Geometry check sheet. Reference: drawing and pictorial views, mm from the part's lowest x, y, z. A direction names the side the tool comes from. Round coordinates to 2 decimals unless told otherwise and drop trailing zeros. Write each loop counter-clockwise with the first axis right and the second up, starting at its lowest first coordinate (ties: lowest second). Pieces come first, ordered by that corner, then holes. Notation, with made-up numbers: (14, -33) -> (65, -33) arc R22 cw to (65, -2) -> close; hole circle Ø11 at (58.5, 53). An arc over 180 degrees is marked (long way). Answer as a JSON object with one key per item and string values. Group by question number.
(1) Sectioned sample at B-B on y = 19.05. Record the cut outline in (x, z).
(2) Set-up check for the marked faces 1, 2 and 3: record each of +Z, -Z, +X, -X, +Y, -Y from which the full face is reachable in a straight line by a thin tool's end or side.
(3) Scan lines: L1, parallel to X at y = 8, z = 8 (1 decimal); L2, parallel to Y at x = 5, z = 30 (1 decimal); L3, parallel to Y at x = 5.5, z = 27.5. Record each from-to range of solid material in increasing order. Write a range as from..to.
(4) Gauge pin test, flat ends, axial feed: pin 1 Ø4.5 at (y, z) = (4.5, 28) entering from +X (1 decimal); pin 2 Ø2 at (y, z) = (6.06, 41.02) entering from -X; pin 3 Ø2.5 at (x, z) = (7, 23.5) entering from +Y; pin 4 Ø3 at (y, z) = (26, 19) entering from +X. Record the tip position at first contact, or that the pin passes through.
(5) Sectioned sample at D-D on y = 31. Record the cut outline in (x, z) (1 decimal).
(6) Sectioned sample at C-C on x = 6.75. Record the cut outline in (y, z) (1 decimal), and give its area (3 significant figures).
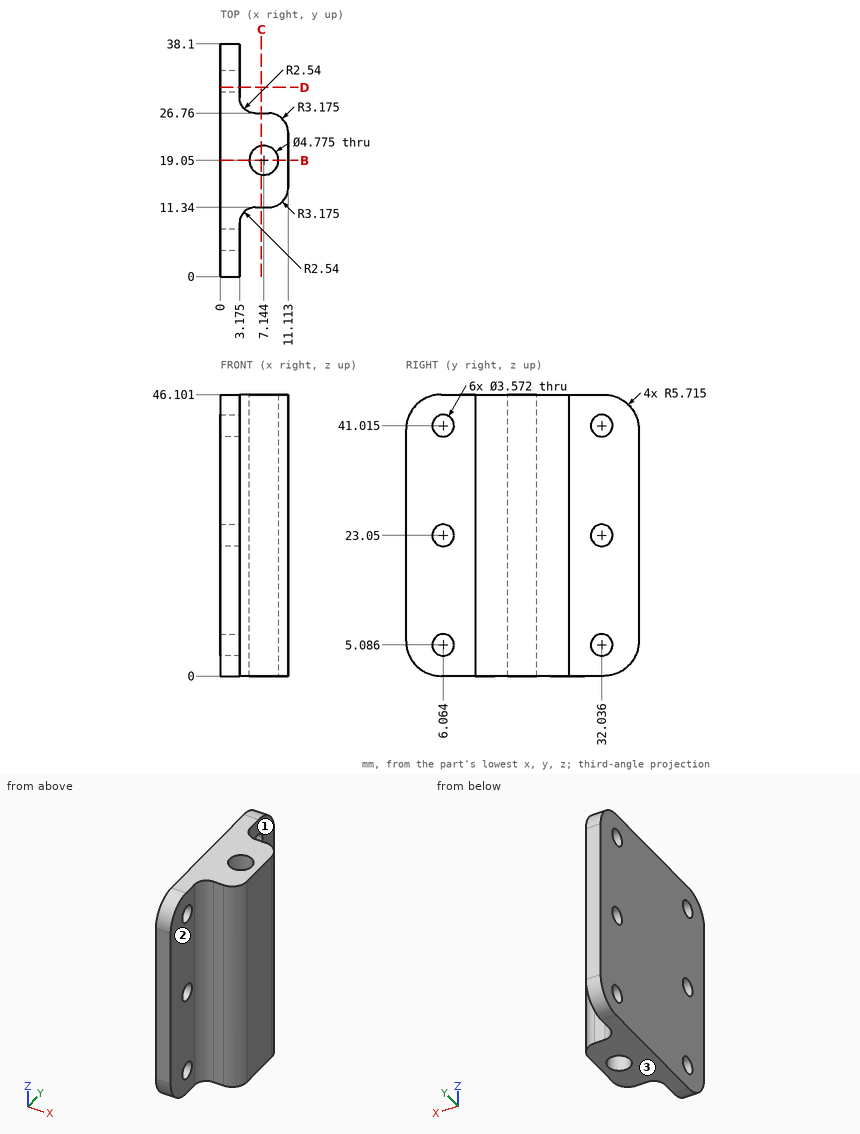
Computed values:
{
 "1": {"outline": "(0, 0) -> (4.76, 0) -> (4.76, 46.1) -> (0, 46.1) -> close; (9.53, 0) -> (11.11, 0) -> (11.11, 46.1) -> (9.53, 46.1) -> close"},
 "2": {"face 1": "+Z, -Z, +X, +Y", "face 2": "+Z, -Z, +X, -Y", "face 3": "-Z, +X, -X, +Y, -Y"},
 "3": {"L1": "0..3.2", "L2": "11.2..18, 20.1..26.9", "L3": "11.33..17.32, 20.78..26.77"},
 "4": {"pin 1": "x = 3.2", "pin 2": "through", "pin 3": "y = 26.76", "pin 4": "x = 10.98"},
 "5": {"outline": "(0, 0) -> (3.2, 0) -> (3.2, 3.6) -> (0, 3.6) -> close; (0, 6.5) -> (3.2, 6.5) -> (3.2, 21.6) -> (0, 21.6) -> close; (0, 24.5) -> (3.2, 24.5) -> (3.2, 39.6) -> (0, 39.6) -> close; (0, 42.5) -> (3.2, 42.5) -> (3.2, 46.1) -> (0, 46.1) -> close"},
 "6": {"outline": "(11.3, 0) -> (16.7, 0) -> (16.7, 46.1) -> (11.3, 46.1) -> close; (21.4, 0) -> (26.8, 0) -> (26.8, 46.1) -> (21.4, 46.1) -> close", "area": "494 mm2"}
}
